```python
from build123d import *

# Parameters (mm, degrees)
SKETCH_1_W               = 76
SKETCH_1_H               = 31
SKETCH_1_W_2             = 66
SKETCH_1_H_2             = 21
EXTRUDE_1_DEPTH          = 19
SKETCH_3_W               = 76
SKETCH_3_H               = 31
SKETCH_3_R               = 4
SKETCH_3_W_2             = 8
SKETCH_3_H_2             = 22.5
EXTRUDE_3_DEPTH          = 5
FILLET_1_R               = 2
FILLET_2_R               = 2
CUT_EXTRUDE_2_DEPTH      = 46.224440295
CUT_EXTRUDE_2_DEPTH_BACK = 46.224440295
SKETCH_5_W               = 76.758909218
SKETCH_5_H               = 3.977461231
SKETCH_6_W               = 76
SKETCH_6_H               = 24
EXTRUDE_4_DEPTH          = 12.177461231
SKETCH_8_R               = 2.3
CUT_EXTRUDE_5_DEPTH      = 58.806920001
SKETCH_13_W              = 65.911954831
SKETCH_13_H              = 1.022538769
CUT_EXTRUDE_6_DEPTH      = 19
SKETCH_14_R              = 4
CUT_EXTRUDE_7_DEPTH      = 4


with BuildPart() as part:
    # 草圖1 → 填料-伸長1 (new body)
    with BuildSketch(Plane(origin=(0, 0, 0), x_dir=(1, 0, 0), z_dir=(0, 1, 0))):
        Rectangle(SKETCH_1_W, SKETCH_1_H)
        Rectangle(SKETCH_1_W_2, SKETCH_1_H_2, mode=Mode.SUBTRACT)
    extrude(amount=EXTRUDE_1_DEPTH)

    # 草圖3 → 填料-伸長3 (add)
    with BuildSketch(Plane(origin=(0, 0, 0), x_dir=(1, 0, 0), z_dir=(0, 1, 0))):
        Rectangle(SKETCH_3_W, SKETCH_3_H)
        with Locations(Location((-21.8, 0, 0), (0, 0, 270))):
            Circle(SKETCH_3_R, mode=Mode.SUBTRACT)
        with Locations((27, 0.75)):
            Rectangle(SKETCH_3_W_2, SKETCH_3_H_2, mode=Mode.SUBTRACT)
    extrude(amount=-EXTRUDE_3_DEPTH)

    # 圓角1
    fillet_1_edges = [part.edges().sort_by_distance(p)[0] for p in [
        (-21.8, 0, -4),
    ]]
    fillet(fillet_1_edges, radius=FILLET_1_R)

    # 圓角2
    fillet_2_edges = [part.edges().sort_by_distance(p)[0] for p in [
        (23, 0, 0),
    ]]
    fillet(fillet_2_edges, radius=FILLET_2_R)

    # 草圖5 → 除料-伸長2 (cut, two sides: drawn at the far end of the back side and taken through both)
    with BuildSketch(Plane(origin=(0, 0, 0), x_dir=(1, 0, 0), z_dir=(0, 1, 0)).offset(-CUT_EXTRUDE_2_DEPTH_BACK)):
        with Locations((0.379454609, -13.511269385)):
            Rectangle(SKETCH_5_W, SKETCH_5_H)
    extrude(amount=CUT_EXTRUDE_2_DEPTH + CUT_EXTRUDE_2_DEPTH_BACK, mode=Mode.SUBTRACT)

    # 草圖6 → 填料-伸長4 (add)
    with BuildSketch(Plane.XY.offset(-27.677461231)):
        with Locations((0, 7)):
            Rectangle(SKETCH_6_W, SKETCH_6_H)
    extrude(amount=EXTRUDE_4_DEPTH)

    # 草圖8 → 除料-伸長5 (cut, through all)
    with BuildSketch(Plane.XY.offset(-27.677461231)):
        with Locations((19.287892817, 6.851763466)):
            Circle(SKETCH_8_R)
        with Locations(Location((-19.287892817, 6.851763466, 0), (0, 0, 180))):
            Circle(SKETCH_8_R)
    extrude(amount=CUT_EXTRUDE_5_DEPTH, mode=Mode.SUBTRACT)

    # 草圖13 → 除料-伸長6 (cut)
    with BuildSketch(Plane(origin=(0, 19, 0), x_dir=(1, 0, 0), z_dir=(0, 1, 0))):
        with Locations((-0.044022584, -11.011269385)):
            Rectangle(SKETCH_13_W, SKETCH_13_H)
    extrude(amount=-CUT_EXTRUDE_6_DEPTH, mode=Mode.SUBTRACT)

    # 草圖14 → 除料-伸長7 (cut)
    with BuildSketch(Plane.XY.offset(-10.5)):
        with Locations((-19.287892817, 6.851763466)):
            Circle(SKETCH_14_R)
        with Locations((19.287892817, 6.851763466)):
            Circle(SKETCH_14_R)
    extrude(amount=-CUT_EXTRUDE_7_DEPTH, mode=Mode.SUBTRACT)


solid = part.part
```
Read the model definition and answer for the solid it produces. Units are mm, in the model's axes. A direction names the side the tool comes from. Coordinates: 2 decimals unless noted, no trailing zeros. Write each loop counter-clockwise with the first axis right and the second up, starting at its lowest first coordinate (ties: lowest second). Pieces come first, ordered by that corner, then holes. Notation, with made-up numbers: (21, -21) -> (36, -21) arc R23 ccw to (36, 6) -> close; hole circle Ø5 at (76, 78.25). An arc over 180 degrees is marked (long way). Return JSON: item names as keys, results as strings.
1. Determine the mould class of faces 6 (the face through (22.4, -0.57, -0.15)), 7 (the face through (-19, 4, -14.5)), 8 (the face through (27, 0, -11)), 9 (the face through (-16.99, 6.75, -21.18)) for opening direction Y: pulls with the +Y half, pulls with the -Y half, needs draft (parallel to the pull), parting line crosses it, or undercut.
Found:
{"face 6": "pulls with the +Y half", "face 7": "undercut", "face 8": "pulls with the -Y half", "face 9": "undercut"}
2. A cutting plane is placed at D-D (y = 13.75). Determine the outline of the cut face in (x, z), and give its area (3 significant figures).
Found:
{"outline": "(-38, -27.68) -> (38, -27.68) -> (38, 11.52) -> (32.91, 11.52) -> (32.91, 10.5) -> (33, 10.5) -> (33, -10.5) -> (-33, -10.5) -> (-33, 11.52) -> (-38, 11.52) -> close", "area": "1,530 mm2"}
3. A cutting plane is placed at B-B (y = 8). Determine the outline of the cut face in (x, z).
Found:
{"outline": "(-38, -27.68) -> (-21.28, -27.68) -> (-21.28, -14.5) -> (-23.12, -14.5) -> (-23.12, -10.5) -> (-33, -10.5) -> (-33, 11.52) -> (-38, 11.52) -> close; (-17.3, -27.68) -> (17.3, -27.68) -> (17.3, -14.5) -> (15.46, -14.5) -> (15.46, -10.5) -> (-15.46, -10.5) -> (-15.46, -14.5) -> (-17.3, -14.5) -> close; (21.28, -27.68) -> (38, -27.68) -> (38, 11.52) -> (32.91, 11.52) -> (32.91, 10.5) -> (33, 10.5) -> (33, -10.5) -> (23.12, -10.5) -> (23.12, -14.5) -> (21.28, -14.5) -> close"}
4. A cutting plane is placed at C-C (z = -7). Determine the outline of the cut face in (x, y), and give its area (3 significant figures).
Found:
{"outline": "(-38, -5) -> (23, -5) -> (23, -2) arc R2 ccw to (21, 0) -> (-33, 0) -> (-33, 19) -> (-38, 19) -> close; (31, -5) -> (38, -5) -> (38, 19) -> (33, 19) -> (33, 0) -> (31, 0) -> close", "area": "529 mm2"}
5. A tool of negligible diameter and unlimited length cuts with its end or side. For faces 1 (the face through (23, -4, -1)), 2 (the face through (-33, 10, 1)), 3 (the face through (33, 9, 0)), 4 (the face through (16.99, 6.95, -21.18)), 5 (the face through (16.34, 9.555, -12.472)), from which of +Z, -Z, +X, -X, +Y, -Y can it reach the whole face along a straight path? Write none if from no direction.
Found:
{"face 1": "-Y", "face 2": "+Z, +Y", "face 3": "+Y", "face 4": "+Z, -Z", "face 5": "+Z"}
6. A cutting plane is placed at A-A (z = 0). Determine the outline of the cut face in (x, y), and give its area (3 significant figures).
Found:
{"outline": "(-38, -5) -> (-25.8, -5) -> (-25.8, -2) arc R2 ccw to (-27.8, 0) -> (-33, 0) -> (-33, 19) -> (-38, 19) -> close; (-17.8, -5) -> (23, -5) -> (23, -2) arc R2 ccw to (21, 0) -> (-15.8, 0) arc R2 ccw to (-17.8, -2) -> close; (31, -5) -> (38, -5) -> (38, 19) -> (33, 19) -> (33, 0) -> (31, 0) -> close", "area": "487 mm2"}
7. Find the intervals of material crossed by line 1 along X through (y, z) = (14.5, 3); line 2 along X through (y, z) = (-3, -2); line 3 along X through (y, z) = (-0.5, -3), in increasing order. Write a range as from..to.
Found:
{"line 1": "-38..-33, 33..38", "line 2": "-38..-25.26, -18.34..23, 31..38", "line 3": "-38..-25.39, -18.21..22.32, 31..38"}
8. Each of these flat-tipped pins is pushed along its axis until it touches: P1, Ø2.5, axis at x = 20.5, y = 7.5, coming from the +Z side; P2, Ø5.5, axis at x = 19.29, y = 6.85, coming from the -Z side; P3, Ø4, axis at x = -29.5, y = 14, coming from the +Z side; P4, Ø1.2, axis at x = 28.5, z = -11, coming from the -Y side. Where does it stop, or does it pass through?
Found:
{"P1": "z = -14.5", "P2": "z = -27.68", "P3": "z = -10.5", "P4": "y = 0"}
